Work out the finished part from the listing and answer in its coordinate system (mm). Coordinates: 2 decimals unless noted, no trailing zeros. Order: outer loops, then holes, each group sorted by start corner. A loop starts at its lowest first (then second) coordinate and runs counter-clockwise, first axis right, second up.
1. Determine the mould class of faces 1 (the flat face through (5, 0, -197)), 2 (the flat face through (0.5, 5.1, 0)), 3 (the flat face through (5, 10, -197)) for opening direction Y: +Y half, -Y half, draft (parallel to the pull), parting line (faces both ways), or undercut.
2. A flat-ended cylindrical pin translates along its axis: pin 1 Ø2.5 at (y, z) = (5, -390) entering from +X. Find the tip coordinate at first contact, or state that the pin passes through.
3. The part is cut by section B-B, the plane x = 3.75. Give the vertices of the cut face in (y, z).
4. The part is cut by section A-A, the plane z = -334.5. Give the vertices of the cut face in (x, y).
5. The part is cut by section C-C, the plane y = 5. Count the separate pieces of the cut face and the enclosed holes in it, then the cut area to 3 significant figures.
6. Find the intervals of material crossed by probe 1 along Y at (x, z) = (4.75, -100); probe 2 along Y at (x, z) = (9.3, -10), in increasing order.
```python
from build123d import *

# Parameters (mm, degrees)
SKETCH1_W           = 10
SKETCH1_H           = 10
SKETCH1_W_2         = 8
SKETCH1_H_2         = 8
BOSS_EXTRUDE1_DEPTH = 400
FILLET1_R           = 1
SKETCH2_R           = 2
CUT_EXTRUDE1_DEPTH  = 27


with BuildPart() as part:
    # Sketch1 → Boss-Extrude1 (new body)
    with BuildSketch(Plane.XY):
        with Locations((5, 5)):
            Rectangle(SKETCH1_W, SKETCH1_H)
        with Locations((5, 5)):
            Rectangle(SKETCH1_W_2, SKETCH1_H_2, mode=Mode.SUBTRACT)
    extrude(amount=-BOSS_EXTRUDE1_DEPTH)

    # Fillet1
    fillet1_edges = [part.edges().sort_by_distance(p)[0] for p in [
        (1, 1, -200),
        (1, 9, -200),
        (9, 9, -200),
        (9, 1, -200),
        (0, 10, -200),
        (10, 10, -200),
        (10, 0, -200),
        (0, 0, -200),
    ]]
    fillet(fillet1_edges, radius=FILLET1_R)

    # Sketch2 → Cut-Extrude1 (cut)
    with BuildSketch(Plane(origin=(10, 0, 0), x_dir=(0, 0, -1), z_dir=(1, 0, 0))):
        with Locations((200, 5)):
            Circle(SKETCH2_R)
        with Locations((225, 5)):
            Circle(SKETCH2_R)
        with Locations((175, 5)):
            Circle(SKETCH2_R)
        with Locations((10, 5)):
            Circle(SKETCH2_R)
        with Locations((35, 5)):
            Circle(SKETCH2_R)
        with Locations((390, 5)):
            Circle(SKETCH2_R)
        with Locations((365, 5)):
            Circle(SKETCH2_R)
    extrude(amount=-CUT_EXTRUDE1_DEPTH, mode=Mode.SUBTRACT)


solid = part.part
```
Geometry says:
1. face 1: -Y half
1. face 2: draft
1. face 3: +Y half
2. pin 1: passes through
3. outline: (0, -400) - (1, -400) - (1, 0) - (0, 0) - close; (9, -400) - (10, -400) - (10, 0) - (9, 0) - close
4. outline: (0, 1) arc R1 ccw to (1, 0) - (9, 0) arc R1 ccw to (10, 1) - (10, 9) arc R1 ccw to (9, 10) - (1, 10) arc R1 ccw to (0, 9) - close; hole (1, 2) arc R1 ccw to (2, 1) - (8, 1) arc R1 ccw to (9, 2) - (9, 8) arc R1 ccw to (8, 9) - (2, 9) arc R1 ccw to (1, 8) - close
5. separate pieces: 16
5. enclosed holes: 0
5. area: 744 mm2
6. probe 1: y = 0 to 1, 9 to 10
6. probe 2: y = 0.05 to 3, 7 to 9.95
